Autodesk Inventor part; units mm, degrees
ref_plane "YZ Plane" through (0, 0, 0) normal (1, 0, 0) x (0, 1, 0)
ref_plane "XZ Plane" through (0, 0, 0) normal (0, 1, 0) x (-1, 0, 0)
ref_plane "XY Plane" through (0, 0, 0) normal (0, 0, 1) x (1, 0, 0)
sketch "Sketch1" plane through (0, 0, 0) normal (0, 1, 0) x (-1, 0, 0)
  line L0 (4.0415, 0) -> (2.0207, -3.5)
  line L1 (2.0207, -3.5) -> (-2.0207, -3.5)
  line L2 (-2.0207, -3.5) -> (-4.0415, 0)
  line L3 (-4.0415, 0) -> (-2.0207, 3.5)
  line L4 (-2.0207, 3.5) -> (2.0207, 3.5)
  line L5 (2.0207, 3.5) -> (4.0415, 0)
  point P0 (0, 0)
  point P1 (0, 0)
  dimension "d0" = 7
extrude "Extrusion1" add sketch "Sketch1" along normal blind 16
sketch "Sketch2" plane through (0, 0, 0) normal (0, -1, 0) x (1, 0, 0)
  circle A0 centre (0, 0) radius 2
  dimension "d3" = 4
extrude "Extrusion2" add sketch "Sketch2" along normal blind 5
sketch "Sketch3" plane through (0, 16, 0) normal (0, 1, 0) x (1, 0, 0)
  circle A0 centre (0, 0) radius 2
  dimension "d6" = 4
extrude "Extrusion3" cut sketch "Sketch3" against normal blind 5
properties part number "dystans 20mm"
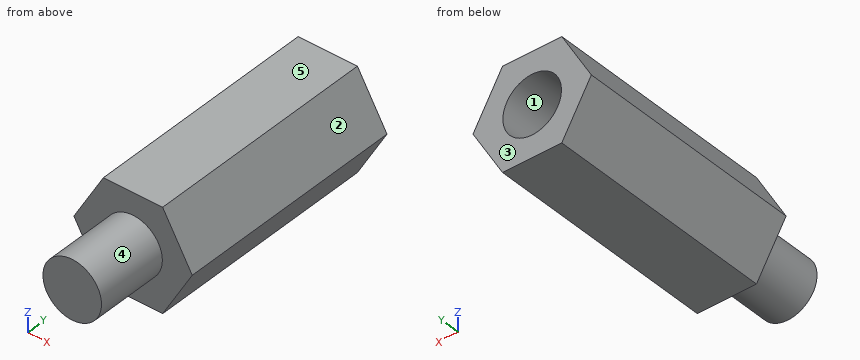
For this review, take the finished solid that the model builds, in its own axes (mm). Face numbers are marked on the shaded views. A direction names the side the tool comes from. Round coordinates to 2 decimals unless told otherwise and drop trailing zeros. Loops run counter-clockwise (first coordinate to the right, second up) from the corner with the lowest first, then second, coordinate; pieces in that order, holes last.
Q1. Add section B-B on y = 13.75. Write out the cut boundary in (x, z), plus the area to 3 significant figures.
Result sheet:
outline: (-4.04, 0) - (-2.02, -3.5) - (2.02, -3.5) - (4.04, 0) - (2.02, 3.5) - (-2.02, 3.5) - close; hole circle Ø4 at (0, 0)
area: 29.9 mm2
Q2. Mouldability with a two-part tool opening along X and no side actions: class the marked faces 1, 2 and 3 as +X half, -X half, draft (parallel to the pull), parting line (faces both ways), or undercut.
Result sheet:
face 1: undercut
face 2: +X half
face 3: draft
Q3. Machinability: for the marked faces 4 and 5, which of the approach directions +Z, -Z, +X, -X, +Y, -Y give a long, thin tool a straight path to every point of the face, cutting with its end or side? Answer none if there is none.
Result sheet:
face 4: -Y
face 5: +Z, +X, -X, +Y, -Y
Q4. Add section C-C on y = 0.5. Write out the cut boundary in (x, z).
Result sheet:
outline: (-4.04, 0) - (-2.02, -3.5) - (2.02, -3.5) - (4.04, 0) - (2.02, 3.5) - (-2.02, 3.5) - close
Q5. Add section A-A on x = 0. Write out the cut boundary in (y, z), plus the area to 3 significant figures.
Result sheet:
outline: (-5, -2) - (0, -2) - (0, -3.5) - (16, -3.5) - (16, -2) - (11, -2) - (11, 2) - (16, 2) - (16, 3.5) - (0, 3.5) - (0, 2) - (-5, 2) - close
area: 112 mm2
Q6. To check wall thickness, follow line 1 along Z through (x, y) = (0, 14.6); line 2 along Y through (x, z) = (2.5, 0.25); line 3 along X through (y, z) = (11.5, -1.75). State the ranges of each line that lie inside material, in increasing order.
Result sheet:
line 1: z = -3.5 to -2, 2 to 3.5
line 2: y = 0 to 16
line 3: x = -3.03 to -0.97, 0.97 to 3.03
Q7. Add section D-D on z = -1. Write out the cut boundary in (x, y), plus the area to 3 significant figures.
Result sheet:
outline: (-3.46, 0) - (-1.73, 0) - (-1.73, -5) - (1.73, -5) - (1.73, 0) - (3.46, 0) - (3.46, 16) - (1.73, 16) - (1.73, 11) - (-1.73, 11) - (-1.73, 16) - (-3.46, 16) - close
area: 111 mm2
Q8. Insertion check: pin 1 Ø2 at (x, z) = (-0.5, -0.5) entering from +Y; pin 2 Ø2 at (y, z) = (6, 2.5) entering from +X. Each pin has a flat end and moves straight along its axis. Give the tip position at first contact, or say it passes through.
Result sheet:
pin 1: stops at y = 11
pin 2: stops at x = 3.18
